Autodesk Inventor part; units mm, degrees
ref_plane "YZ Plane" through (0, 0, 0) normal (1, 0, 0) x (0, 1, 0)
ref_plane "XZ Plane" through (0, 0, 0) normal (0, 1, 0) x (-1, 0, 0)
ref_plane "XY Plane" through (0, 0, 0) normal (0, 0, 1) x (1, 0, 0)
sketch "Sketch1" plane through (0, 0, 0) normal (0, 1, 0) x (-1, 0, 0)
  line L0 (0, 0) -> (49.25, 0)
  line L1 (49.25, 0) -> (49.25, -39.75)
  line L2 (49.25, -39.75) -> (0, -39.75)
  line L3 (0, -39.75) -> (0, 0)
  line L4 (49.25, 0) -> (37.75, 0)
  line L5 (37.75, 0) -> (37.75, -10)
  line L6 (37.75, -10) -> (18.75, -10)
  line L7 (0, 0) -> (12, 0)
  line L8 (12, 0) -> (18.75, -10)
  line L9 (49.25, -19.875) -> (61.5731, -19.875)
  line L10 (37.75, -39.75) -> (37.75, -29.75)
  line L11 (37.75, -29.75) -> (18.75, -29.75)
  line L12 (12, -39.75) -> (18.75, -29.75)
  dimension "d0" = 49.25
  dimension "d1" = 39.75
  dimension "d2" = 11.5
  dimension "d3" = 10
  dimension "d4" = 19
  dimension "d5" = 12
extrude "Extrusion1" add sketch "Sketch1" along normal blind 15 contours L0 L8 L6 L5 L1 L2 L10 L11 L12 L3
chamfer "Chamfer1" distance 5 angle 15 1 edges at (-28.25, 15, -10) measured on face at (-31.4167, 5, -10)
chamfer "Chamfer2" distance 5 angle 15 1 edges at (-15.375, 15, -5) measured on face at (-14.25, 8.3333, -3.3333)
chamfer "Chamfer3" distance 5 angle 15 1 edges at (-37.75, 15, -5) measured on face at (-37.75, 8.3333, -3.3333)
chamfer "Chamfer4" distance 5 angle 15 1 edges at (-37.75, 0, -5) measured on face at (-37.75, 3.3333, -3.3333)
chamfer "Chamfer5" distance 5 angle 15 1 edges at (-28.25, 0, -10) measured on face at (-25.0833, 5, -10)
chamfer "Chamfer6" distance 5 angle 15 1 edges at (-15.375, 0, -5) measured on face at (-14.25, 5, -3.3333)
chamfer "Chamfer7" distance 5 angle 15 1 edges at (-28.25, 15, -29.75) measured on face at (-25.0833, 5, -29.75)
chamfer "Chamfer8" distance 5 angle 15 1 edges at (-15.375, 15, -34.75) measured on face at (-14.25, 8.3333, -36.4167)
chamfer "Chamfer9" distance 5 angle 15 1 edges at (-15.375, 0, -34.75) measured on face at (-14.25, 6.6667, -36.4167)
chamfer "Chamfer10" distance 5 angle 15 1 edges at (-28.25, 0, -29.75) measured on face at (-31.4167, 5, -29.75)
chamfer "Chamfer11" distance 5 angle 15 1 edges at (-37.75, 15, -34.75) measured on face at (-37.75, 8.3333, -36.4167)
chamfer "Chamfer12" distance 5 angle 15 1 edges at (-37.75, 0, -34.75) measured on face at (-37.75, 5.0002, -36.4167)
sketch "Sketch2" plane through (-49.25, 0, -39.75) normal (-1, 0, 0) x (0, 0, 1)
  line L0 (39.75, 0) -> (0, 0)
  line L1 (19.875, 0) -> (7.175, 0)
  line L2 (7.175, 0) -> (32.575, 0)
  line L3 (32.575, 0) -> (32.575, 15)
  line L4 (28.4103, 15) -> (39.75, 15)
  line L5 (32.575, 7.5) -> (32.575, 3)
  line L6 (32.575, 3) -> (32.575, 12)
  line L7 (7.175, 0) -> (7.175, 15)
  line L8 (32.575, 12) -> (7.175, 12)
  line L9 (7.175, 12) -> (7.175, 3)
  line L10 (7.175, 3) -> (32.575, 3)
  line L11 (32.575, 3) -> (32.575, 12)
  point P0 (7.175, 12)
  dimension "d44" = 12.7
  dimension "d45" = 25.4
  dimension "d46" = 4.5
  dimension "d47" = 9
extrude "Extrusion2" add sketch "Sketch2" along normal blind 6 contours L10 L7 L8 L3
chamfer "Chamfer13" distance 5 angle 10 1 edges at (-52.25, 3, -32.575) measured on face at (-51.25, 9, -32.575)
chamfer "Chamfer14" distance 5 angle 10 1 edges at (-52.25, 3, -7.175) measured on face at (-51.25, 6, -7.175)
sketch "Sketch3" plane through (-49.25, 0, -39.75) normal (-1, 0, 0) x (0, 0, 1)
  line L0 (39.75, 0) -> (39.75, 15)
  line L1 (39.75, 7.5) -> (36.25, 7.5)
  line L2 (0, 15) -> (39.75, 15)
  line L3 (19.875, 15) -> (19.875, 18.5612)
  circle A0 centre (36.25, 7.5) radius 1.35
  circle A1 centre (3.5, 7.5) radius 1.35
  dimension "d56" = 3.5
  dimension "d57" = 2.7
extrude "Extrusion3" add sketch "Sketch3" along normal blind 3.8
properties part number "vga_plug"
Verification items for the finished model (mm, model axes). A direction names the side the tool comes from. Round coordinates to 2 decimals unless told otherwise and drop trailing zeros. Loops run counter-clockwise (first coordinate to the right, second up) from the corner with the lowest first, then second, coordinate; pieces in that order, holes last. Notation, with made-up numbers: (18.5, 36.5) -> (51.5, 36.5) arc R16 ccw to (51.5, 48.5) -> close; hole circle Ø5 at (50.25, -23.5). An arc over 180 degrees is marked (long way). Answer as a JSON object with one key per item and string values.
Q1. Section check C-C (x = -37). Record the boundary of the cut face in (y, z).
Data:
{"outline": "(0, -28.41) -> (5, -29.75) -> (10, -29.75) -> (15, -28.41) -> (15, -11.34) -> (10, -10) -> (5, -10) -> (0, -11.34) -> close"}
Q2. Section check A-A (x = -51). Record the boundary of the cut face in (y, z) (3 decimals), then the cut area to 3 significant figures.
Data:
{"outline": "(3, -31.693) -> (8, -32.575) -> (12, -32.575) -> (12, -7.175) -> (8, -7.175) -> (3, -8.057) -> close; circle Ø2.7 at (7.5, -36.25); circle Ø2.7 at (7.5, -3.5)", "area": "236 mm2"}
Q3. Go/stop test with flat-tipped pins: P1, Ø5, axis at x = -53.5, z = -25, coming from the +Y side; P2, Ø0.8, axis at y = 7.5, z = -36, coming from the -X side; P3, Ø1.5, axis at x = -22, y = 12.5, coming from the +Z side. Record where each tip stops, or that it passes through.
Data:
{"P1": "stops at y = 12", "P2": "stops at x = -53.05", "P3": "stops at z = -10.47"}
Q4. Access from +Z, -Z, +X, -X, +Y, -Y to the whole of each face (thin tool, end or side, straight path). Record for faces 1 (the flat face through (-38.43, 12.54, -5.75)), 2 (the flat face through (-15.33, 7.46, -4.93)), 3 (the flat face through (-52.208, 5.465, -7.622)).
Data:
{"face 1": "+Z, +Y", "face 2": "+Z, +Y, -Y", "face 3": "-X, -Y"}
Q5. Scan lines: line 1 (Z direction, x = -20.5, y = 7); line 2 (X direction, y = 0.75, z = -12); line 3 (X direction, y = 1.75, z = -10.5). Record each from-to range of solid material in increasing order. Write a range as from..to.
Data:
{"line 1": "z = -29.75..-10", "line 2": "x = -49.25..0", "line 3": "x = -49.25..-38.62, -18.04..0"}
Q6. Section check D-D (y = 4.25). Record the boundary of the cut face in (x, z).
Data:
{"outline": "(-55.25, -31.91) -> (-49.25, -31.91) -> (-49.25, -39.75) -> (-37.95, -39.75) -> (-37.95, -29.55) -> (-18.64, -29.55) -> (-11.76, -39.75) -> (0, -39.75) -> (0, 0) -> (-11.76, 0) -> (-18.64, -10.2) -> (-37.95, -10.2) -> (-37.95, 0) -> (-49.25, 0) -> (-49.25, -7.84) -> (-55.25, -7.84) -> close"}
Q7. Draft check along Z on faces 4 (the flat face through (-52.208, 5.465, -32.128)), 5 (the flat face through (-14.81, 12.54, -34.37)), 6 (the cylindrical face through (-51.123, 6.362, -35.524)), 7 (the flat face through (-52, 3, -20)). Enter one of: pulls with the +Z half, pulls with the -Z half, needs draft (parallel to the pull), parting line crosses it, or undercut.
Data:
{"face 4": "undercut", "face 5": "pulls with the -Z half", "face 6": "undercut", "face 7": "needs draft"}
Q8. Section check B-B (z = -36). Record the boundary of the cut face in (x, y), then the cut area to 3 significant figures.
Data:
{"outline": "(-53.05, 6.17) -> (-49.25, 6.17) -> (-49.25, 0) -> (-39.09, 0) -> (-37.75, 5) -> (-37.75, 10) -> (-39.09, 15) -> (-49.25, 15) -> (-49.25, 8.83) -> (-53.05, 8.83) -> close; (-14.53, 5) -> (-12.91, 0) -> (0, 0) -> (0, 15) -> (-12.91, 15) -> (-14.53, 10) -> close", "area": "386 mm2"}
